```python
from build123d import *

# Parameters (mm, degrees)
CROQUIS1_R              = 12.5
SALIENTE_EXTRUIR1_DEPTH = 24
CROQUIS2_W              = 9.4
CROQUIS2_H              = 17.525
CORTAR_EXTRUIR1_DEPTH   = 18
CROQUIS3_W              = 9.2
CROQUIS3_H              = 17.9
SALIENTE_EXTRUIR2_DEPTH = 5
CHAFL_N1_SIZE           = 1
CHAFL_N2_SIZE           = 1
CROQUIS4_R              = 1.9
CORTAR_EXTRUIR2_DEPTH   = 34.963215395
CHAFL_N3_SIZE           = 1
CROQUIS5_W              = 6
CROQUIS5_H              = 14
CORTAR_EXTRUIR3_DEPTH   = 26.228951623
CHAFL_N4_SIZE           = 1.7
CHAFL_N5_SIZE           = 0.5
CHAFL_N6_SIZE           = 0.5


with BuildPart() as part:
    # Croquis1 → Saliente-Extruir1 (new body)
    with BuildSketch(Plane.XY):
        Circle(CROQUIS1_R)
    extrude(amount=SALIENTE_EXTRUIR1_DEPTH)

    # Croquis2 → Cortar-Extruir1 (cut)
    with BuildSketch(Plane.XY.offset(24)):
        Rectangle(CROQUIS2_W, CROQUIS2_H)
    extrude(amount=-CORTAR_EXTRUIR1_DEPTH, mode=Mode.SUBTRACT)

    # Croquis3 → Saliente-Extruir2 (add)
    with BuildSketch(Plane(origin=(0, 0, 0), x_dir=(-1, 0, 0), z_dir=(0, 0, -1))):
        Rectangle(CROQUIS3_W, CROQUIS3_H)
    extrude(amount=SALIENTE_EXTRUIR2_DEPTH)

    # Chaflán1
    chafl_n1_edges = [part.edges().sort_by_distance(p)[0] for p in [
        (-4.6, 0, -5),
        (0, 8.95, -5),
        (4.6, 0, -5),
        (0, -8.95, -5),
    ]]
    chamfer(chafl_n1_edges, length=CHAFL_N1_SIZE)

    # Chaflán2
    chafl_n2_edges = [part.edges().sort_by_distance(p)[0] for p in [
        (-12.5, 0, 0),
    ]]
    chamfer(chafl_n2_edges, length=CHAFL_N2_SIZE)

    # Croquis4 → Cortar-Extruir2 (cut, through all)
    with BuildSketch(Plane.XY.offset(24)):
        with Locations((-7.875, 0)):
            Circle(CROQUIS4_R)
        with Locations((7.875, 0)):
            Circle(CROQUIS4_R)
    extrude(amount=-CORTAR_EXTRUIR2_DEPTH, mode=Mode.SUBTRACT)

    # Chaflán3
    chafl_n3_edges = [part.edges().sort_by_distance(p)[0] for p in [
        (-12.5, 0, 24),
    ]]
    chamfer(chafl_n3_edges, length=CHAFL_N3_SIZE)

    # Croquis5 → Cortar-Extruir3 (cut, through all)
    with BuildSketch(Plane.XY.offset(6)):
        Rectangle(CROQUIS5_W, CROQUIS5_H)
    extrude(amount=-CORTAR_EXTRUIR3_DEPTH, mode=Mode.SUBTRACT)

    # Chaflán4
    chafl_n4_edges = [part.edges().sort_by_distance(p)[0] for p in [
        (4.7, 0, 6),
        (0, -8.7625, 6),
        (-4.7, 0, 6),
        (0, 8.7625, 6),
    ]]
    chamfer(chafl_n4_edges, length=CHAFL_N4_SIZE - 0.0001)  # a hair under: the kernel refuses the full size

    # Chaflán5
    chafl_n5_edges = [part.edges().sort_by_distance(p)[0] for p in [
        (-9.775, 0, 24),
        (5.975, 0, 24),
    ]]
    chamfer(chafl_n5_edges, length=CHAFL_N5_SIZE)

    # Chaflán6
    chafl_n6_edges = [part.edges().sort_by_distance(p)[0] for p in [
        (0, -8.7625, 24),
        (4.7, 0, 24),
        (0, 8.7625, 24),
        (-4.7, 0, 24),
    ]]
    chamfer(chafl_n6_edges, length=CHAFL_N6_SIZE)


solid = part.part
```
Work out the finished part from the listing and answer in its coordinate system (mm). A direction names the side the tool comes from. Round coordinates to 2 decimals unless told otherwise and drop trailing zeros. Loops run counter-clockwise (first coordinate to the right, second up) from the corner with the lowest first, then second, coordinate; pieces in that order, holes last.
(1) The part is cut by section C-C, the plane y = 0. Give the number of separate pieces and of enclosed holes in the cut face, and give its area (3 significant figures).
Computed values:
separate pieces: 4
enclosed holes: 0
area: 228 mm2
(2) The part is cut by section B-B, the plane x = 0. Give the vertices of the cut face in (y, z), and give its area (3 significant figures).
Computed values:
outline: (-12.5, 1) - (-11.5, 0) - (-8.95, 0) - (-8.95, -4) - (-7.95, -5) - (-7, -5) - (-7, 6) - (-7.06, 6) - (-8.76, 7.7) - (-8.76, 23.5) - (-9.26, 24) - (-11.5, 24) - (-12.5, 23) - close; (7, -5) - (7.95, -5) - (8.95, -4) - (8.95, 0) - (11.5, 0) - (12.5, 1) - (12.5, 23) - (11.5, 24) - (9.26, 24) - (8.76, 23.5) - (8.76, 7.7) - (7.06, 6) - (7, 6) - close
area: 220 mm2
(3) The part is cut by section D-D, the plane z = 4.25. Give the vertices of the cut face in (x, y) (3 decimals), and give its area (3 significant figures).
Computed values:
outline: circle Ø25 at (0, 0); hole circle Ø3.8 at (-7.875, 0); hole (-3, -7) - (3, -7) - (3, 7) - (-3, 7) - close; hole circle Ø3.8 at (7.875, 0)
area: 384 mm2
(4) For faces 1 (the flat face through (0, 8.95, -2)), 2 (the flat face through (0, -7, 1)), 3 (the flat face through (0, 8.762, 16)), 4 (the flat face through (-4.6, 0, -2)), determine the directions among +Z, -Z, +X, -X, +Y, -Y from which every point of the face is accessible in a straight line to the end or side of a thin tool.
Computed values:
face 1: -Z, +X, -X, +Y
face 2: +Z, -Z
face 3: +Z
face 4: -Z, -X, +Y, -Y
(5) Each of these flat-tipped pins is pushed along its axis until it touches: P1, Ø3, axis at y = -4, z = -2.5, coming from the +X side; P2, Ø4.5, axis at y = -3.5, z = -3, coming from the -X side; P3, Ø4, axis at x = 6.5, z = 7, coming from the -Y side. Where does it stop, or does it pass through?
Computed values:
P1: stops at x = 4.6
P2: stops at x = -4.6
P3: stops at y = -11.66
(6) The mould has two halves that part along X. Classify faces 5 (the flat face through (4.1, -0.1, -4.5)), 6 (the flat face through (-0.07, 7.9, 6.84)), 7 (the flat face through (5, 0, 0)), 8 (the flat face through (4.7, 0, 16)): pulls with the +X half, pulls with the -X half, needs draft (parallel to the pull), parting line crosses it, or undercut.
Computed values:
face 5: pulls with the +X half
face 6: undercut
face 7: needs draft
face 8: undercut
(7) Find the intervals of material crossed by L1, parallel to Y at x = 0.5, z = -3.25; L2, parallel to X at y = 0.25, z = 5.5; L3, parallel to X at y = 0.5, z = 7.75, in increasing order.
Computed values:
L1: y = -8.95 to -7, 7 to 8.95
L2: x = -12.5 to -9.76, -5.99 to -3, 3 to 5.99, 9.76 to 12.5
L3: x = -12.49 to -9.71, -6.04 to -4.7, 4.7 to 6.04, 9.71 to 12.49
(8) The part is cut by section A-A, the plane z = 20.5. Give the vertices of the cut face in (x, y) (1 decimal).
Computed values:
outline: circle Ø25 at (0, 0); hole circle Ø3.8 at (-7.9, 0); hole (-4.7, -8.8) - (4.7, -8.8) - (4.7, 8.8) - (-4.7, 8.8) - close; hole circle Ø3.8 at (7.9, 0)
